Geometry: see drawing. Coordinates: mm, zero at the bounding-box minimum. Give positions to 0.01 mm unless a question says otherwise; leave off trailing zeros. Write each loop counter-clockwise with the first axis right and the second up, starting at its lowest first coordinate (ties: lowest second). Pieces come first, ordered by that corner, then holes. Notation, with made-up numbers: (86, -8.5) - (101, -8.5) arc R21 ccw to (101, 7.5) - close; hole circle Ø9 at (-2.5, 64.25). An arc over 180 degrees is marked (long way). Use CSV: the item, a comma, the result in double quotes. Start each with the question number.
(1) Section A-A on x = 77.5. Output: boundary loops of the cut face in (y, z) (1 decimal).
(2) Line query: probe 1 along Z at (x, y) = (18, 1.5) (1 decimal); probe 2 along Z at (x, y) = (20.5, 7) (1 decimal). Output: solid intervals per line, ascending. Write a range as [from, to].
(3) Section C-C on y = 19.5. Output: boundary loops of the cut face in (x, z) (1 decimal).
(4) First-contact query: pin 1 Ø1.6 at (y, z) = (1.5, 36.5) entering from -X; pin 2 Ø3.5 at (y, z) = (11, 1) entering from +X (1 decimal); pin 3 Ø3.5 at (y, z) = (9, 1) entering from -X. Flat tips, straight axial feed; report the tip coordinate or a pass-through.
(5) Section B-B on z = 26.5. Output: boundary loops of the cut face in (x, y) (1 decimal), and give its area (3 significant figures).
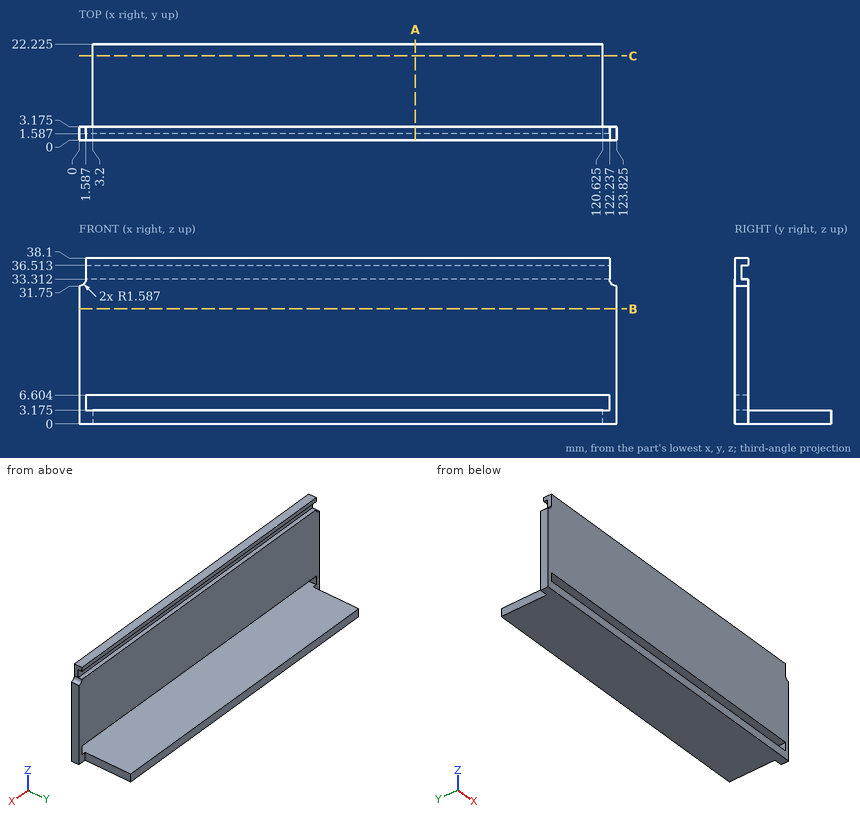
Check values:
1,outline,"(0, 0) - (22.2, 0) - (22.2, 3.2) - (0, 3.2) - close; (0, 6.6) - (3.2, 6.6) - (3.2, 33.3) - (1.6, 33.3) - (1.6, 36.5) - (3.2, 36.5) - (3.2, 38.1) - (0, 38.1) - close"
2,probe 1,"z = [0, 3.2], [6.6, 38.1]"
2,probe 2,"z = [0, 3.2]"
3,outline,"(3.2, 0) - (120.6, 0) - (120.6, 3.2) - (3.2, 3.2) - close"
4,pin 1,"stops at x = 1.59"
4,pin 2,"stops at x = 120.6"
4,pin 3,"stops at x = 3.2"
5,outline,"(0, 0) - (123.8, 0) - (123.8, 3.2) - (0, 3.2) - close"
5,area,"393 mm²"
